Read the model definition and answer for the solid it produces. Units are mm, in the model's axes. Give positions to 0.01 mm unless a question says otherwise; leave off trailing zeros. Write each loop counter-clockwise with the first axis right and the second up, starting at its lowest first coordinate (ties: lowest second). Pieces come first, ordered by that corner, then holes. Notation, with made-up numbers: (79, -19.5) - (134, -19.5) arc R22 cw to (134, -10.5) - close; hole circle Ø10 at (0.5, 4.25). An arc over 180 degrees is marked (long way). Answer as CSV lines item,"result".
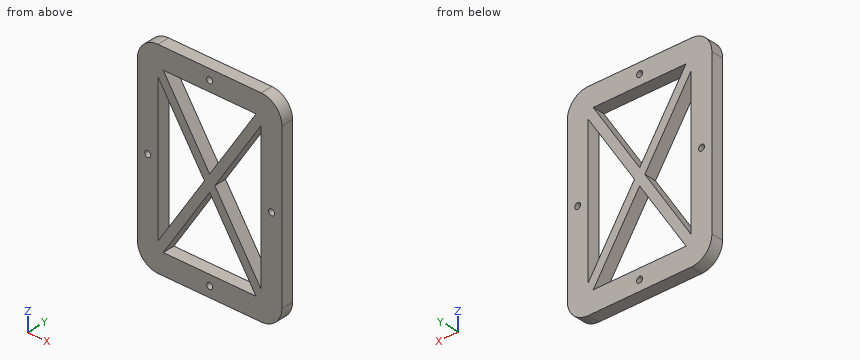
```python
from build123d import *

# Parameters (mm, degrees)
SKETCH1_R           = 1.45
BOSS_EXTRUDE1_DEPTH = 5.85


with BuildPart() as part:
    # Sketch1 → Boss-Extrude1 (new body)
    with BuildSketch(Plane(origin=(0, 0, 0), x_dir=(1, 0, 0), z_dir=(0, 1, 0))):
        with BuildLine():
            ThreePointArc((-25, 49), (-32.071067812, 46.071067812), (-35, 39))
            Line((-35, 39), (-35, -39))
            ThreePointArc((-35, -39), (-32.071067812, -46.071067812), (-25, -49))
            Line((-25, -49), (25, -49))
            ThreePointArc((25, -49), (32.071067812, -46.071067812), (35, -39))
            Line((35, -39), (35, 39))
            ThreePointArc((35, 39), (32.071067812, 46.071067812), (25, 49))
            Line((25, 49), (-25, 49))
        make_face()
        Polygon((-22.5, -39), (0, -3.9), (22.5, -39), align=None, mode=Mode.SUBTRACT)
        Polygon((25, -35.1), (2.5, 0), (25, 35.1), align=None, mode=Mode.SUBTRACT)
        Polygon((22.5, 39), (0, 3.9), (-22.5, 39), align=None, mode=Mode.SUBTRACT)
        Polygon((-25, 35.1), (-2.5, 0), (-25, -35.1), align=None, mode=Mode.SUBTRACT)
        with Locations(Location((0, -44, 0), (0, 0, 270))):
            Circle(SKETCH1_R, mode=Mode.SUBTRACT)
        with Locations(Location((-30, 0, 0), (0, 0, 270))):
            Circle(SKETCH1_R, mode=Mode.SUBTRACT)
        with Locations(Location((0, 44, 0), (0, 0, 270))):
            Circle(SKETCH1_R, mode=Mode.SUBTRACT)
        with Locations(Location((30, 0, 0), (0, 0, 270))):
            Circle(SKETCH1_R, mode=Mode.SUBTRACT)
    extrude(amount=BOSS_EXTRUDE1_DEPTH)


solid = part.part
```
(1) This flat-tipped pin is pushed along its axis until it touches: P1, Ø2.5, axis at x = -30, z = 0, coming from the -Y side. Where does it stop, or does it pass through?
Worked out:
P1,"passes through"
(2) Find the intervals of material crossed by L1, parallel to X at y = 3.65, z = 0; L2, parallel to X at y = 2.95, z = 8; L3, parallel to X at y = 2.65, z = -2, in increasing order.
Worked out:
L1,"x = -35 to -31.45, -28.55 to -25, -2.5 to 2.5, 25 to 28.55, 31.45 to 35"
L2,"x = -35 to -25, -7.63 to -2.63, 2.63 to 7.63, 25 to 35"
L3,"x = -35 to -25, -3.78 to 3.78, 25 to 35"
(3) A cutting plane is placed at A-A (x = 12). Write down the section's boundary in (y, z), and give its area (3 significant figures).
Worked out:
outline,"(0, -49) - (5.85, -49) - (5.85, -39) - (0, -39) - close; (0, -22.62) - (5.85, -22.62) - (5.85, -14.82) - (0, -14.82) - close; (0, 14.82) - (5.85, 14.82) - (5.85, 22.62) - (0, 22.62) - close; (0, 39) - (5.85, 39) - (5.85, 49) - (0, 49) - close"
area,"208 mm^2"
(4) A cutting plane is placed at D-D (x = -30). Write down the section's boundary in (y, z), and give its area (3 significant figures).
Worked out:
outline,"(0, -47.66) - (5.85, -47.66) - (5.85, -1.45) - (0, -1.45) - close; (0, 1.45) - (5.85, 1.45) - (5.85, 47.66) - (0, 47.66) - close"
area,"541 mm^2"
(5) A cutting plane is placed at C-C (y = 2.1). Count the separate pieces of the cut face and the enclosed holes in it, and give its area (3 significant figures).
Worked out:
separate pieces,"1"
enclosed holes,"8"
area,"3,590 mm^2"
(6) A cutting plane is placed at B-B (z = -7.5). Write down the section's boundary in (x, y), and give its area (4 significant figures).
Worked out:
outline,"(-35, 0) - (-25, 0) - (-25, 5.85) - (-35, 5.85) - close; (-7.31, 0) - (-2.31, 0) - (-2.31, 5.85) - (-7.31, 5.85) - close; (2.31, 0) - (7.31, 0) - (7.31, 5.85) - (2.31, 5.85) - close; (25, 0) - (35, 0) - (35, 5.85) - (25, 5.85) - close"
area,"175.5 mm^2"
